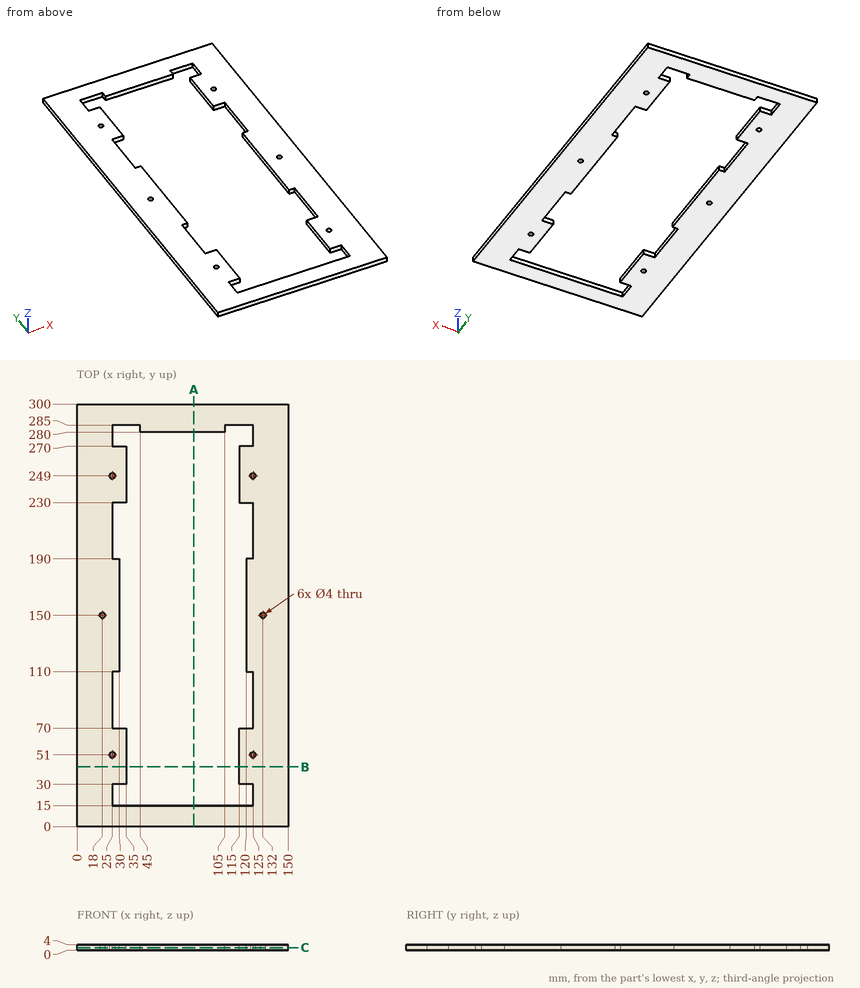
Answer from the drawing. Dimensions are ordinates in mm from the lowest x, y and z of the part. Coordinates: 2 decimals unless noted, no trailing zeros. Loops run counter-clockwise (first coordinate to the right, second up) from the corner with the lowest first, then second, coordinate; pieces in that order, holes last.
Q1. The part is cut by section C-C on z = 1.85. Give the number of separate pieces and of enclosed holes in the cut face, and give its area (3 significant figures).
Q2. The part is cut by section A-A on x = 83. Write down the section's boundary in (y, z).
Q3. The part is cut by section B-B on y = 42.5. Write down the section's boundary in (x, z).
Q4. Consider probe 1 along X at (y, z) = (150, 1.45); probe 2 along X at (y, z) = (51, 1.3); probe 3 along X at (y, z) = (173, 0.35). Determine where each line is inside the solid, lowest interval first.
Results below:
1. separate pieces: 1
1. enclosed holes: 7
1. area: 20,600 mm2
2. outline: (0, 0) - (15, 0) - (15, 4) - (0, 4) - close; (280, 0) - (300, 0) - (300, 4) - (280, 4) - close
3. outline: (0, 0) - (35, 0) - (35, 4) - (0, 4) - close; (115, 0) - (150, 0) - (150, 4) - (115, 4) - close
4. probe 1: x = 0 to 16, 20 to 30, 120 to 130, 134 to 150
4. probe 2: x = 0 to 23, 27 to 35, 115 to 123, 127 to 150
4. probe 3: x = 0 to 30, 120 to 150
